Part print with two shaded views. Sizes in mm from the minimum x, y, z corner. A direction names the side the tool comes from. Coordinates: 2 decimals unless noted, no trailing zeros. Order: outer loops, then holes, each group sorted by start corner. A loop starts at its lowest first (then second) coordinate and runs counter-clockwise, first axis right, second up.
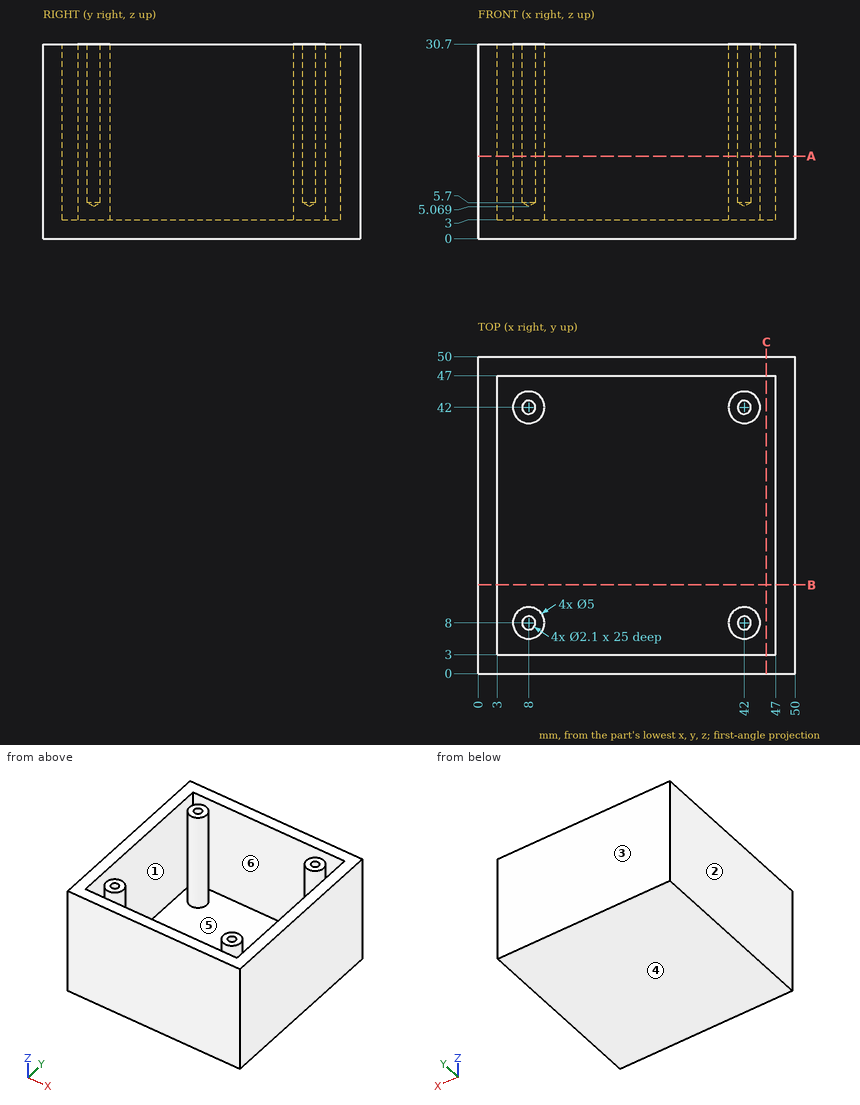
Q1. Pin check, flat tips, straight feed: pin 1 Ø8.5 at (x, z) = (35, 21.5) entering from -Y; pin 2 Ø22 at (x, y) = (26, 20) entering from +Z; pin 3 Ø1.9 at (x, y) = (8, 8) entering from +Z; pin 4 Ø1.3 at (x, y) = (42, 8) entering from +Z. Stop position of each tip, or through.
Results list:
pin 1: stops at y = 0
pin 2: stops at z = 3
pin 3: stops at z = 5.64
pin 4: stops at z = 5.46
Q2. Mould opens along Y. For the marked faces 3, 4, 5 and 6 say: pulls with the +Y half, pulls with the -Y half, needs draft (parallel to the pull), parting line crosses it, or undercut.
Results list:
face 3: pulls with the +Y half
face 4: needs draft
face 5: undercut
face 6: undercut
Q3. Cut at B-B on y = 14. Write the cut outline in (x, z).
Results list:
outline: (0, 0) - (50, 0) - (50, 30.7) - (47, 30.7) - (47, 3) - (3, 3) - (3, 30.7) - (0, 30.7) - close
Q4. Which spindle directions (+Z, -Z, +X, -X, +Y, -Y) get a long thin tool onto all of the face, cutting with end or side? Do the marked faces 1 and 2. Say none if no direction does.
Results list:
face 1: +Z
face 2: +Z, -Z, -X, +Y, -Y
Q5. Cut at A-A on z = 13. Count the separate pieces of the cut face and the enclosed holes in it, and give its area (3 significant figures).
Results list:
separate pieces: 5
enclosed holes: 5
area: 629 mm2
Q6. Wall check: line 1 along Y through (x, z) = (8, 15); line 2 along Y through (x, z) = (31.5, 17). Give the ranges that are in metal, low to high.
Results list:
line 1: y = 0 to 3, 5.5 to 6.95, 9.05 to 10.5, 39.5 to 40.95, 43.05 to 44.5, 47 to 50
line 2: y = 0 to 3, 47 to 50
